```python
from build123d import *

# Parameters (mm, degrees)
F1_DEPTH = 18.9484
F3_DEPTH = 1.143
F4_R     = 0.8382
F5_W     = 11.43
F5_H     = 12.5984
F6_DEPTH = 8.3058
F8_D     = 4.572


with BuildPart() as f1:
    # F0 (on Front) → F1 (new body)
    with BuildSketch(Plane.XZ):
        Polygon((0, 26.304375), (-12.0142, 26.304375), (-12.0142, 8.778375), (-10.2616, 8.778375), (-10.2616, 11.673975), (-7.1374, 11.673975), (-7.1374, 8.778375), (-1.245109, -6.297331), (0, -8.341225), align=None)
    extrude(amount=F1_DEPTH)

    # F2 (on face) → F3 (join)
    with BuildSketch(Plane.XY.offset(26.304375)):
        Polygon((6.0198, 2.1082), (-14.7066, 2.1082), (-14.7066, -23.2918), (-7.414963, -23.2918), (-7.414963, -39.116), (6.0198, -39.116), align=None)
    extrude(amount=F3_DEPTH)

    # F4
    f4_edges = [f1.edges().sort_by_distance(p)[0] for p in [
        (-12.0142, -9.4742, 8.778375),
        (-10.2616, -9.4742, 8.778375),
    ]]
    fillet(f4_edges, radius=F4_R)

    # F5 (on face) → F6 (cut)
    with BuildSketch(Plane(origin=(-12.0142, 0, 0), x_dir=(0, -1, 0), z_dir=(-1, 0, 0))):
        with Locations((5.715, 20.005175)):
            Rectangle(F5_W, F5_H)
    extrude(amount=-F6_DEPTH, mode=Mode.SUBTRACT)

    # F8 (through all)
    with Locations(Plane(origin=(-3.7084, 0, 0), x_dir=(0, -1, 0), z_dir=(-1, 0, 0))):
        with Locations((6.35, 18.430375)):
            Hole(F8_D / 2)


solid = f1.part
```
The listing builds one solid part. Answer for the finished solid, in the listing's coordinates (mm). A direction names the side the tool comes from. Round coordinates to 2 decimals unless told otherwise and drop trailing zeros. Order: outer loops, then holes, each group sorted by start corner. A loop starts at its lowest first (then second) coordinate and runs counter-clockwise, first axis right, second up. Notation, with made-up numbers: (-4, 88) - (26, 88) arc R22 cw to (26, 119) - close; hole circle Ø5 at (56, -38.5). An arc over 180 degrees is marked (long way). Put each result on its own line as item: value. Start each with the question number.
(1) Find section B-B (y = -16). Give the vertices of the cut face in (x, z), plus the area to 3 significant figures.
(2) Find section A-A (y = -6.35). Give the vertices of the cut face in (x, z).
(3) Determine the mould class of faces 5 (the cylindrical face through (-1.828, -8.164, 17.039)), 6 (the flat face through (-4, -18, 27.447)), 7 (the flat face through (-11, -23.292, 27)), 8 (the flat face through (-3, 0, 9)) for opening direction Y: released by +Y, released by -Y, zero draft, split by the parting line, or undercut.
(4) For faces 1 (the flat face through (-12.014, -14, 16)), 2 (the flat face through (2, -18, 26.304)), 3 (the flat face through (-7.137, -9, 10)), 4 (the flat face through (-8, -6, 13.706)), determine the directions among +Z, -Z, +X, -X, +Y, -Y from which every point of the face is accessible in a straight line to the end or side of a thin tool.
(5) Find section D-D (z = 22). Give the vertices of the cut face in (x, y).
(6) Find section C-C (x = -0.75). Give the vertices of the cut face in (y, z).
(7) Given P1, Ø5.5, axis at y = -6.5, z = 20, coming from the -X side; P2, Ø5, axis at y = -6, z = 7.5, coming from the +X side; P3, Ø4, axis at x = -8.5, z = 4, coming from the -Y side; P4, Ø2.5, axis at y = -10, z = 10, coming from the -X side, each flat-ended and moving along its own axis, determine where each tip first touches the part or whether it passes through.
(8) Straight lines are drawn through the part: probe 1 along Y at (x, z) = (-0.75, 18.5); probe 2 along X at (y, z) = (-9, 10.5); probe 3 along Y at (x, z) = (-11.5, 21). For each, find the intervals that lie inside material, in ascending order. Write a range as from..to.
Reply:
1. outline: (-14.71, 26.3) - (-12.01, 26.3) - (-12.01, 9.62) arc R0.84 ccw to (-11.18, 8.78) - (-11.1, 8.78) arc R0.84 ccw to (-10.26, 9.62) - (-10.26, 11.67) - (-7.14, 11.67) - (-7.14, 8.78) - (-1.25, -6.3) - (0, -8.34) - (0, 26.3) - (6.02, 26.3) - (6.02, 27.45) - (-14.71, 27.45) - close
1. area: 289 mm^2
2. outline: (-14.71, 26.3) - (-3.71, 26.3) - (-3.71, 20.72) - (0, 20.72) - (0, 26.3) - (6.02, 26.3) - (6.02, 27.45) - (-14.71, 27.45) - close; (-12.01, 9.62) arc R0.84 ccw to (-11.18, 8.78) - (-11.1, 8.78) arc R0.84 ccw to (-10.26, 9.62) - (-10.26, 11.67) - (-7.14, 11.67) - (-7.14, 8.78) - (-1.25, -6.3) - (0, -8.34) - (0, 16.14) - (-3.71, 16.14) - (-3.71, 13.71) - (-12.01, 13.71) - close
3. face 5: undercut
3. face 6: zero draft
3. face 7: released by -Y
3. face 8: released by +Y
4. face 1: -Z, -X, +Y, -Y
4. face 2: none
4. face 3: -Z, +Y, -Y
4. face 4: -X, +Y
5. outline: (-12.01, -18.95) - (0, -18.95) - (0, 0) - (-3.71, 0) - (-3.71, -11.43) - (-12.01, -11.43) - close
6. outline: (-39.12, 26.3) - (-18.95, 26.3) - (-18.95, -7.11) - (0, -7.11) - (0, 26.3) - (2.11, 26.3) - (2.11, 27.45) - (-39.12, 27.45) - close; hole circle Ø4.57 at (-6.35, 18.43)
7. P1: x = -3.71
7. P2: x = 0
7. P3: through
7. P4: x = -12.01
8. probe 1: -18.95..-8.63, -4.07..0
8. probe 2: -12.01..-10.26, -7.14..0
8. probe 3: -18.95..-11.43
